Print and shaded views of the part. All mm, measured from the part's lowest x, y and z. A direction names the side the tool comes from. Round coordinates to 2 decimals unless told otherwise and drop trailing zeros. Loops run counter-clockwise (first coordinate to the right, second up) from the corner with the lowest first, then second, coordinate; pieces in that order, holes last. Notation, with made-up numbers: (0, -30.5) - (22, -30.5) arc R8 cw to (22, -20.5) - close; hole circle Ø1 at (1.25, 81). An arc over 180 degrees is marked (long way). Put each result on its own line as item: value. Start each with the question number.
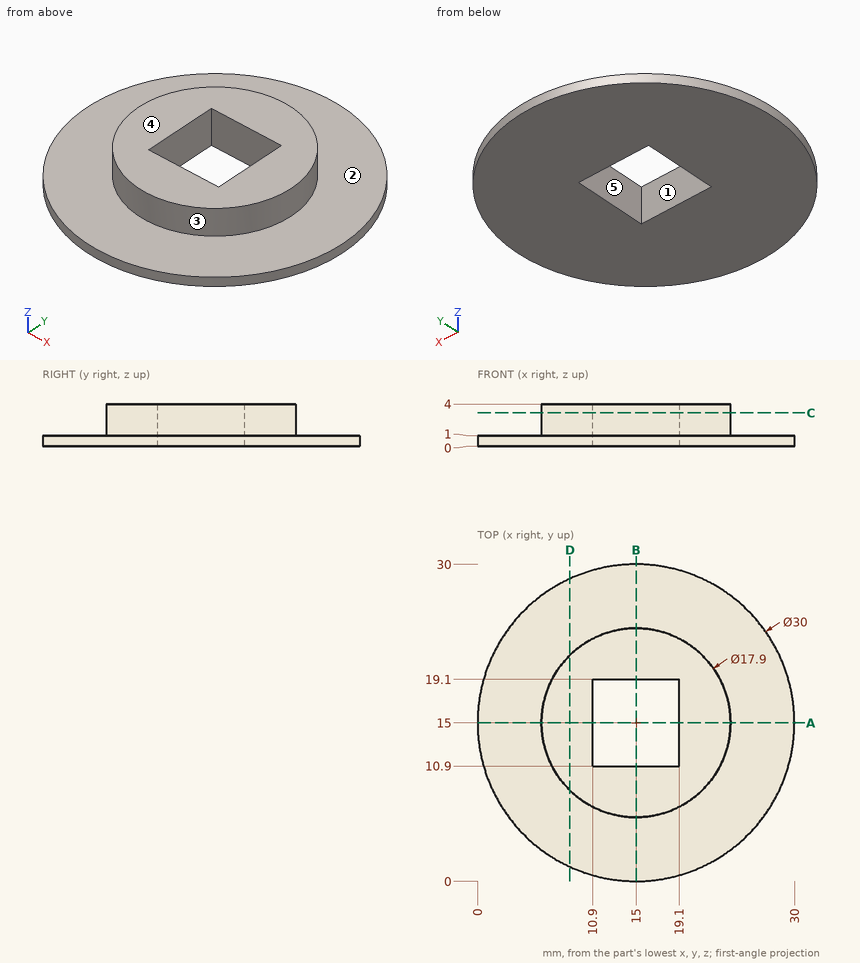
Item 1: Which spindle directions (+Z, -Z, +X, -X, +Y, -Y) get a long thin tool onto all of the face, cutting with end or side? Do the marked faces 4 and 5. Say none if no direction does.
Item 2: Drill centre lines: probe 1 along Y at (x, z) = (15.5, 3.1); probe 2 along X at (y, z) = (16.5, 1.4); probe 3 along Z at (x, y) = (18, 28.5). Where is each one in solid material? Low to high. Write a range as [from, to].
Item 3: Slice it at C-C (z = 3.15). Give the cut face in (x, y), plus the area to 3 significant figures.
Item 4: Slice it at D-D (x = 8.75). Give the cut face in (y, z).
Item 5: Two-plate mould, pull along X, no slides. Class the marked faces 1, 2 and 3: pulls with the +X half, pulls with the -X half, needs draft (parallel to the pull), parting line crosses it, or undercut.
Item 6: Drop flat-ended pins along their axis: pin 1 Ø2 at (y, z) = (17.5, 0.5) entering from -X; pin 2 Ø1.2 at (x, z) = (13, 2.5) entering from -Y; pin 3 Ø2 at (y, z) = (16, 2.5) entering from +X. Give the stop position or say it passes through.
Item 7: Slice it at A-A (y = 15). Give the cut face in (x, z).
Computed values:
1. face 4: +Z, +X, -X, +Y, -Y
1. face 5: +Z, -Z
2. probe 1: y = [6.06, 10.9], [19.1, 23.94]
2. probe 2: x = [6.18, 10.9], [19.1, 23.82]
2. probe 3: z = [0, 1]
3. outline: circle Ø17.9 at (15, 15); hole (10.9, 10.9) - (19.1, 10.9) - (19.1, 19.1) - (10.9, 19.1) - close
3. area: 184 mm^2
4. outline: (1.36, 0) - (28.64, 0) - (28.64, 1) - (21.41, 1) - (21.41, 4) - (8.59, 4) - (8.59, 1) - (1.36, 1) - close
5. face 1: undercut
5. face 2: needs draft
5. face 3: parting line crosses it
6. pin 1: stops at x = 0.08
6. pin 2: stops at y = 6.16
6. pin 3: stops at x = 23.95
7. outline: (0, 0) - (10.9, 0) - (10.9, 4) - (6.05, 4) - (6.05, 1) - (0, 1) - close; (19.1, 0) - (30, 0) - (30, 1) - (23.95, 1) - (23.95, 4) - (19.1, 4) - close
